Study the drawing (mm; zero at the part's minimum x, y, z) and answer. A direction names the side the tool comes from. Give positions to 0.01 mm unless a question says otherwise; leave off trailing zeros. Order: outer loops, then holes, each group sorted by start corner. A loop starts at its lowest first (then second) coordinate and runs counter-clockwise, first axis right, second up. Notation, with made-up numbers: (35.25, 36.25) -> (93.25, 36.25) arc R14 ccw to (93.25, 59.25) -> close; hole circle Ø11 at (63.5, -27). An arc over 180 degrees is marked (long way). Answer as CSV lines item,"result". Start each with the question number.
1. Find the intervals of material crossed by L1, parallel to Z at x = 16, y = 0.7 (1 decimal); L2, parallel to X at y = 1.8, z = 19.5; L3, parallel to X at y = 1.55, z = 14.5, in increasing order.
2. A cutting plane is placed at A-A (x = 27). Give the vertices of the cut face in (y, z) (1 decimal).
3. For a pull along Z with two mould halves and no side action, classify the marked faces 1, 2 and 3 as released by +Z, released by -Z, zero draft, split by the parting line, or undercut.
4. For the marked faces 4, 5, 6 and 7, determine the directions among +Z, -Z, +X, -X, +Y, -Y from which every point of the face is accessible in a straight line to the end or side of a thin tool.
5. Flat-ended cylindrical pins translate along their axes: pin 1 (1.8 mm diameter, centred on x = 30.07, z = 14.62, fed in from +Y); pin 2 (0.9 mm diameter, centred on y = 1.5, z = 25.5, fed in from +X); pin 3 (1.5 mm diameter, centred on x = 29, y = 1, fed in from -Z). Find the tip coordinate at first contact, or state that the pin passes through.
6. A cutting plane is placed at D-D (x = 16). Give the vertices of the cut face in (y, z) (1 decimal).
7. A cutting plane is placed at C-C (y = 1.05). State how many separate pieces and enclosed holes the cut face has, then the cut area to 3 significant figures.
8. A cutting plane is placed at B-B (z = 5.5). Give the vertices of the cut face in (x, y).
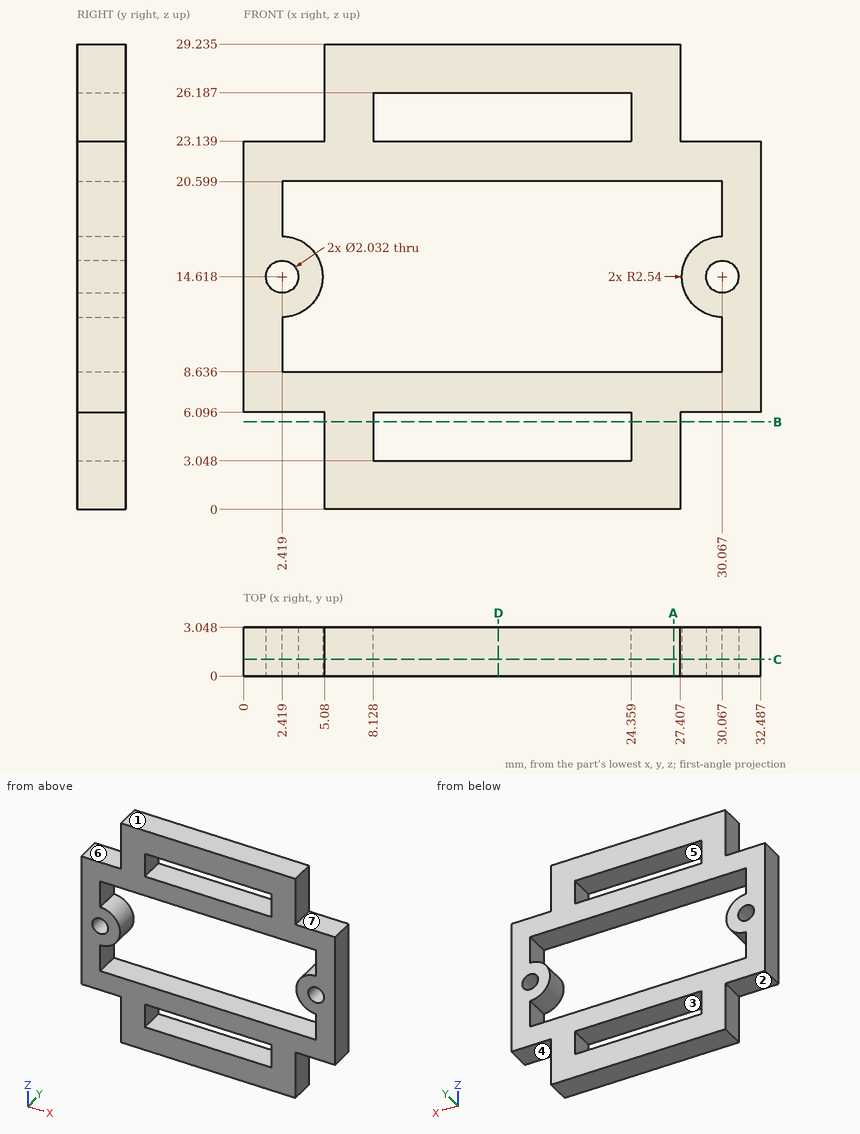
Answer sheet:
1,L1,"z = 0 to 3, 6.1 to 8.6, 20.6 to 23.1, 26.2 to 29.2"
1,L2,"x = 0 to 2.42, 30.07 to 32.49"
1,L3,"x = 0 to 1.41, 3.43 to 4.96, 27.53 to 29.06, 31.08 to 32.49"
2,outline,"(0, 0) -> (3, 0) -> (3, 8.6) -> (0, 8.6) -> close; (0, 20.6) -> (3, 20.6) -> (3, 29.2) -> (0, 29.2) -> close"
3,face 1,"released by +Z"
3,face 2,"released by -Z"
3,face 3,"undercut"
4,face 4,"-Z, +X, +Y, -Y"
4,face 5,"+Y, -Y"
4,face 6,"+Z, -X, +Y, -Y"
4,face 7,"+Z, +X, +Y, -Y"
5,pin 1,"passes through"
5,pin 2,"stops at x = 27.41"
5,pin 3,"stops at z = 6.1"
6,outline,"(0, 0) -> (3, 0) -> (3, 3) -> (0, 3) -> close; (0, 6.1) -> (3, 6.1) -> (3, 8.6) -> (0, 8.6) -> close; (0, 20.6) -> (3, 20.6) -> (3, 23.1) -> (0, 23.1) -> close; (0, 26.2) -> (3, 26.2) -> (3, 29.2) -> (0, 29.2) -> close"
7,separate pieces,"1"
7,enclosed holes,"5"
7,area,"410 mm^2"
8,outline,"(5.08, 0) -> (8.13, 0) -> (8.13, 3.05) -> (5.08, 3.05) -> close; (24.36, 0) -> (27.41, 0) -> (27.41, 3.05) -> (24.36, 3.05) -> close"
